Work out the finished part from the listing and answer in its coordinate system (mm). Face numbers are marked on the shaded views. A direction names the side the tool comes from. Coordinates: 2 decimals unless noted, no trailing zeros. Order: outer loops, then holes, each group sorted by start corner. A loop starts at its lowest first (then second) coordinate and runs counter-clockwise, first axis right, second up.
1. Find the intervals of material crossed by probe 1 along Y at (x, z) = (40.5, 5.5); probe 2 along Z at (x, y) = (53.5, -6.25); probe 3 along X at (y, z) = (-21, 18.5), in increasing order.
2. Flat-ended cylindrical pins translate along their axes: pin 1 Ø4 at (y, z) = (-11.5, 17.5) entering from +X; pin 2 Ø4 at (x, y) = (29, -12) entering from +Z. Find the tip coordinate at first contact, or state that the pin passes through.
3. The part is cut by section C-C, the plane z = 5. Give the vertices of the cut face in (x, y).
4. Determine the mould class of the marked faces 4, 5 and 6 for opening direction X: +X half, -X half, draft (parallel to the pull), parting line (faces both ways), or undercut.
5. The part is cut by section A-A, the plane y = -11.5. Give the vertices of the cut face in (x, z).
6. A tool of negligible diameter and unlimited length cuts with its end or side. For the marked faces 1, 2 and 3, from which of +Z, -Z, +X, -X, +Y, -Y can it reach the whole face along a straight path? Write none if from no direction.
7. The part is cut by section B-B, the plane x = 49. Give the vertices of the cut face in (y, z), then the cut area to 3 significant figures.
8. The part is cut by section D-D, the plane z = 28. Give the vertices of the cut face in (x, y).
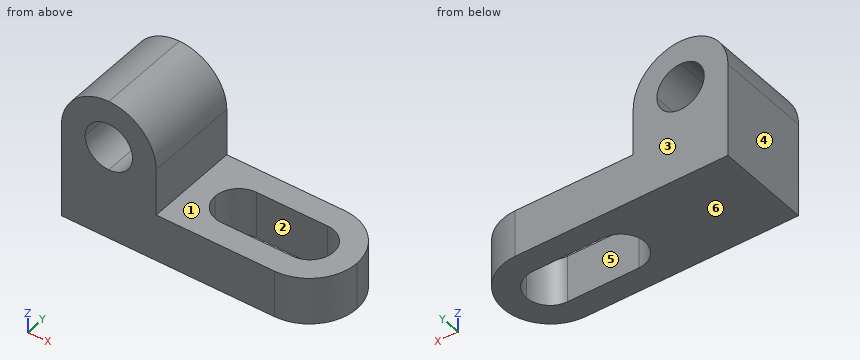
```python
from build123d import *

# Parameters (mm, degrees)
F1_DEPTH = 25.4
F2_DEPTH = 25.4
F4_DEPTH = 25.4


with BuildPart() as f1:
    # F0 (on Front) → F1 (new body)
    with BuildSketch(Plane.XZ):
        with BuildLine():
            Line((0, 25.4), (0, 0))
            Line((0, 0), (12.7, 0))
            Line((12.7, 0), (12.7, 12.7))
            ThreePointArc((12.7, 12.7), (3.7197438789, 16.4197438789), (0, 25.4))
        make_face()
        with BuildLine():
            ThreePointArc((12.7, 38.1), (3.7197438789, 34.3802561211), (0, 25.4))
            Line((0, 25.4), (6.35, 25.4))
            ThreePointArc((6.35, 25.4), (8.2098719395, 29.8901280605), (12.7, 31.75))
            Line((12.7, 31.75), (12.7, 38.1))
        make_face()
        with BuildLine():
            Line((0, 38.1), (0, 25.4))
            ThreePointArc((0, 25.4), (3.7197438789, 34.3802561211), (12.7, 38.1))
            Line((12.7, 38.1), (0, 38.1))
        make_face()
        with BuildLine():
            Line((6.35, 25.4), (0, 25.4))
            ThreePointArc((0, 25.4), (3.7197438789, 16.4197438789), (12.7, 12.7))
            Line((12.7, 12.7), (12.7, 19.05))
            ThreePointArc((12.7, 19.05), (8.2098719395, 20.9098719395), (6.35, 25.4))
        make_face()
        with BuildLine():
            Line((12.7, 12.7), (12.7, 0))
            Line((12.7, 0), (69.85, 0))
            Line((69.85, 0), (69.85, 12.7))
            Line((69.85, 12.7), (25.4, 12.7))
            Line((25.4, 12.7), (25.4, 25.4))
            ThreePointArc((25.4, 25.4), (21.6802561211, 16.4197438789), (12.7, 12.7))
        make_face()
        with BuildLine():
            ThreePointArc((25.4, 25.4), (21.6802561211, 34.3802561211), (12.7, 38.1))
            Line((12.7, 38.1), (12.7, 31.75))
            ThreePointArc((12.7, 31.75), (17.1901280605, 29.8901280605), (19.05, 25.4))
            Line((19.05, 25.4), (25.4, 25.4))
        make_face()
        with BuildLine():
            Line((25.4, 38.1), (12.7, 38.1))
            ThreePointArc((12.7, 38.1), (21.6802561211, 34.3802561211), (25.4, 25.4))
            Line((25.4, 25.4), (25.4, 38.1))
        make_face()
        with BuildLine():
            Line((12.7, 19.05), (12.7, 12.7))
            ThreePointArc((12.7, 12.7), (21.6802561211, 16.4197438789), (25.4, 25.4))
            Line((25.4, 25.4), (19.05, 25.4))
            ThreePointArc((19.05, 25.4), (17.1901280605, 20.9098719395), (12.7, 19.05))
        make_face()
    extrude(amount=F1_DEPTH)

    # F0 (on Front) → F2 (cut)
    with BuildSketch(Plane.XZ):
        with BuildLine():
            Line((0, 38.1), (0, 25.4))
            ThreePointArc((0, 25.4), (3.7197438789, 34.3802561211), (12.7, 38.1))
            Line((12.7, 38.1), (0, 38.1))
        make_face()
        with BuildLine():
            Line((25.4, 38.1), (12.7, 38.1))
            ThreePointArc((12.7, 38.1), (21.6802561211, 34.3802561211), (25.4, 25.4))
            Line((25.4, 25.4), (25.4, 38.1))
        make_face()
    extrude(amount=F2_DEPTH, mode=Mode.SUBTRACT)

    # F3 (on face) → F4 (cut)
    with BuildSketch(Plane.XY.offset(12.7)):
        with BuildLine():
            ThreePointArc((44.45, -12.7), (42.5901280605, -8.2098719395), (38.1, -6.35))
            Line((38.1, -6.35), (38.1, -12.7))
            Line((38.1, -12.7), (44.45, -12.7))
        make_face()
        with BuildLine():
            Line((38.1, -12.7), (38.1, -6.35))
            ThreePointArc((38.1, -6.35), (33.6098719395, -8.2098719395), (31.75, -12.7))
            Line((31.75, -12.7), (38.1, -12.7))
        make_face()
        with BuildLine():
            Line((44.45, -12.7), (38.1, -12.7))
            Line((38.1, -12.7), (38.1, -19.05))
            ThreePointArc((38.1, -19.05), (42.5901280605, -17.1901280605), (44.45, -12.7))
        make_face()
        with BuildLine():
            Line((38.1, -19.05), (38.1, -12.7))
            Line((38.1, -12.7), (31.75, -12.7))
            ThreePointArc((31.75, -12.7), (33.6098719395, -17.1901280605), (38.1, -19.05))
        make_face()
        with BuildLine():
            ThreePointArc((63.5, -12.7), (61.6401280605, -8.2098719395), (57.15, -6.35))
            Line((57.15, -6.35), (57.15, -12.7))
            Line((57.15, -12.7), (63.5, -12.7))
        make_face()
        with BuildLine():
            Line((57.15, -12.7), (57.15, -6.35))
            ThreePointArc((57.15, -6.35), (52.6598719395, -8.2098719395), (50.8, -12.7))
            Line((50.8, -12.7), (57.15, -12.7))
        make_face()
        with BuildLine():
            Line((63.5, -12.7), (57.15, -12.7))
            Line((57.15, -12.7), (57.15, -19.05))
            ThreePointArc((57.15, -19.05), (61.6401280605, -17.1901280605), (63.5, -12.7))
        make_face()
        with BuildLine():
            Line((57.15, -12.7), (50.8, -12.7))
            ThreePointArc((50.8, -12.7), (52.6598719395, -17.1901280605), (57.15, -19.05))
            Line((57.15, -19.05), (57.15, -12.7))
        make_face()
        with BuildLine():
            Line((57.15, -6.35), (38.1, -6.35))
            ThreePointArc((38.1, -6.35), (42.5901280605, -8.2098719395), (44.45, -12.7))
            Line((44.45, -12.7), (50.8, -12.7))
            ThreePointArc((50.8, -12.7), (52.6598719395, -8.2098719395), (57.15, -6.35))
        make_face()
        with BuildLine():
            Line((50.8, -12.7), (44.45, -12.7))
            ThreePointArc((44.45, -12.7), (42.5901280605, -17.1901280605), (38.1, -19.05))
            Line((38.1, -19.05), (57.15, -19.05))
            ThreePointArc((57.15, -19.05), (52.6598719395, -17.1901280605), (50.8, -12.7))
        make_face()
        with BuildLine():
            Line((69.85, -12.7), (69.7292175596, -12.7))
            ThreePointArc((69.7292175596, -12.7), (66.0521098797, -21.6376550953), (57.15, -25.4))
            Line((57.15, -25.4), (69.85, -25.4))
            Line((69.85, -25.4), (69.85, -12.7))
        make_face()
        with BuildLine():
            Line((69.85, 0), (57.15, 0))
            ThreePointArc((57.15, 0), (66.0521098797, -3.7623449047), (69.7292175596, -12.7))
            Line((69.7292175596, -12.7), (69.85, -12.7))
            Line((69.85, -12.7), (69.85, 0))
        make_face()
    extrude(amount=-F4_DEPTH, mode=Mode.SUBTRACT)


solid = f1.part
```
Geometry says:
1. probe 1: y = -25.4 to -19.05, -6.35 to 0
1. probe 2: z = 0 to 12.7
1. probe 3: x = 0 to 25.4
2. pin 1: stops at x = 25.4
2. pin 2: stops at z = 12.7
3. outline: (0, -25.4) - (57.15, -25.4) arc R12.7 ccw to (57.15, 0) - (0, 0) - close; hole (38.1, -19.05) - (57.15, -19.05) arc R6.35 ccw to (57.15, -6.35) - (38.1, -6.35) arc R6.35 ccw to start
4. face 4: -X half
4. face 5: undercut
4. face 6: draft
5. outline: (0, 0) - (31.86, 0) - (31.86, 12.7) - (25.4, 12.7) - (25.4, 25.4) arc R12.7 ccw to (0, 25.4) - close; (63.39, 0) - (69.67, 0) - (69.67, 12.7) - (63.39, 12.7) - close; hole circle Ø12.7 at (12.7, 25.4)
6. face 1: +Z, +X, +Y, -Y
6. face 2: +Z, -Z
6. face 3: +Z, -Z, +X, -X, +Y
7. outline: (-25.4, 0) - (-19.05, 0) - (-19.05, 12.7) - (-25.4, 12.7) - close; (-6.35, 0) - (0, 0) - (0, 12.7) - (-6.35, 12.7) - close
7. area: 161 mm2
8. outline: (0.27, -25.4) - (6.91, -25.4) - (6.91, 0) - (0.27, 0) - close; (18.49, -25.4) - (25.13, -25.4) - (25.13, 0) - (18.49, 0) - close
